Source: CAD feature listing. Evaluate the final solid. Frame: model axes, mm. A direction names the side the tool comes from. Round coordinates to 2 decimals unless told otherwise and drop trailing zeros. Loops run counter-clockwise (first coordinate to the right, second up) from the corner with the lowest first, then second, coordinate; pieces in that order, holes last. Notation, with made-up numbers: (80.25, -27.5) -> (85.25, -27.5) arc R18 cw to (85.25, 4.5) -> close; hole circle Ø3 at (-38, 61.5). An arc over 180 degrees is marked (long way). Return JSON: item names as keys, results as strings. Group by question number.
```python
from build123d import *

# Parameters (mm, degrees)
BOSS_EXTRUDE1_DEPTH = 1.524


with BuildPart() as part:
    # Sketch1 → Boss-Extrude1 (new body)
    with BuildSketch(Plane.XY):
        with BuildLine():
            Line((0, 36.766680051), (1.524, 36.766680051))
            Line((1.524, 36.766680051), (1.524, 38.982585825))
            Line((1.524, 38.982585825), (2.733148625, 38.375210755))
            Line((2.733148625, 38.375210755), (3.173163666, 37.740395602))
            ThreePointArc((3.173163666, 37.740395602), (2.76380149, 34.435260273), (2.111575724, 31.169360935))
            Line((2.111575724, 31.169360935), (3.752142818, 30.122391454))
            Line((3.752142818, 30.122391454), (1.811466825, 29.982342047))
            ThreePointArc((1.811466825, 29.982342047), (0.512131502, 25.907377193), (-1.167502988, 21.973875087))
            ThreePointArc((-1.167502988, 21.973875087), (-1.496079249, 21.518994961), (-1.833336721, 21.070513426))
            Line((-1.833336721, 21.070513426), (-0.732526116, 18.85197433))
            Line((-0.732526116, 18.85197433), (-2.63805659, 20.068036908))
            ThreePointArc((-2.63805659, 20.068036908), (-4.673990558, 17.880915718), (-6.922800397, 15.913333311))
            Line((-6.922800397, 15.913333311), (-6.657550745, 14.318385487))
            Line((-6.657550745, 14.318385487), (-7.787922662, 15.257015862))
            ThreePointArc((-7.787922662, 15.257015862), (-11.338183777, 13.037842353), (-15.16934542, 11.349267359))
            Line((-15.16934542, 11.349267359), (-15.723402455, 8.912532591))
            Line((-15.723402455, 8.912532591), (-16.164329399, 11.013577704))
            ThreePointArc((-16.164329399, 11.013577704), (-19.953116728, 10.084187136), (-23.831985363, 9.668189099))
            ThreePointArc((-23.831985363, 9.668189099), (-24.076075542, 9.604568952), (-24.319524306, 9.538536852))
            Line((-24.319524306, 9.538536852), (-24.695691572, 6.942894819))
            Line((-24.695691572, 6.942894819), (-25.27612991, 9.253711636))
            ThreePointArc((-25.27612991, 9.253711636), (-26.183331796, 8.945243362), (-27.078300937, 8.602901171))
            ThreePointArc((-27.078300937, 8.602901171), (-30.246868295, 7.97926726), (-32.962548086, 6.231748554))
            Line((-32.962548086, 6.231748554), (-32.532162923, 5.243855929))
            Line((-32.532162923, 5.243855929), (-33.480739201, 5.694007752))
            ThreePointArc((-33.480739201, 5.694007752), (-34.200835329, 4.756022574), (-34.785563978, 3.728186482))
            ThreePointArc((-34.785563978, 3.728186482), (-36.445037111, 2.053220727), (-37.942668533, 0.232105276))
            Line((-37.942668533, 0.232105276), (-37.938700484, 2.479305956))
            Line((-37.938700484, 2.479305956), (-35.209054914, 6.010902474))
            Line((-35.209054914, 6.010902474), (-36.41486015, 6.942894819))
            Line((-36.41486015, 6.942894819), (-37.934290003, 4.977067008))
            Line((-37.934290003, 4.977067008), (-37.932464483, 6.010902474))
            ThreePointArc((-37.932464483, 6.010902474), (-36.563778761, 7.575593862), (-34.971875943, 8.912532591))
            ThreePointArc((-34.971875943, 8.912532591), (-32.901550016, 9.116540541), (-30.910632492, 9.719960876))
            Line((-30.910632492, 9.719960876), (-30.910632492, 11.8237405))
            Line((-30.910632492, 11.8237405), (-29.95978759, 10.169722089))
            ThreePointArc((-29.95978759, 10.169722089), (-29.013670421, 10.741179379), (-28.13202331, 11.407812338))
            ThreePointArc((-28.13202331, 11.407812338), (-27.492889702, 11.44249827), (-26.85283117, 11.446965831))
            ThreePointArc((-26.85283117, 11.446965831), (-23.965434713, 11.605929088), (-21.115990345, 12.098873725))
            Line((-21.115990345, 12.098873725), (-20.706404595, 14.318385487))
            Line((-20.706404595, 14.318385487), (-20.019464899, 12.381448288))
            ThreePointArc((-20.019464899, 12.381448288), (-16.437841998, 13.695848714), (-13.099310966, 15.542435195))
            ThreePointArc((-13.099310966, 15.542435195), (-12.585951474, 15.59640554), (-12.076536587, 15.679755638))
            Line((-12.076536587, 15.679755638), (-11.031123121, 17.962204557))
            Line((-11.031123121, 17.962204557), (-11.249347571, 15.880665501))
            ThreePointArc((-11.249347571, 15.880665501), (-7.425610197, 18.149727188), (-5.157240456, 21.973875087))
            ThreePointArc((-5.157240456, 21.973875087), (-4.381951062, 24.278807565), (-3.708542129, 26.615537712))
            Line((-3.708542129, 26.615537712), (-5.157240456, 27.453082135))
            Line((-5.157240456, 27.453082135), (-3.412165634, 27.787336527))
            ThreePointArc((-3.412165634, 27.787336527), (-2.457151359, 32.712229886), (-1.951475295, 37.703313794))
            ThreePointArc((-1.951475295, 37.703313794), (-1.128983902, 38.484354747), (0, 38.375210755))
            Line((0, 38.375210755), (0, 36.766680051))
        make_face()
    extrude(amount=BOSS_EXTRUDE1_DEPTH)


solid = part.part
```
(1) Ray query, line 1 (X direction, y = 22, z = 1.1); line 2 (Y direction, x = -12.5, z = 0.5); line 3 (Y direction, x = -30.5, z = 1.35). Return the intervals inside material, ascending.
(2) Pin query (flat end, axial travel): pin 1 (0.5 mm diameter, centred on y = 38, z = 0.5, fed in from -X); pin 2 (0.8 mm diameter, centred on y = 11, z = 0.5, fed in from -X). Return the tip coordinate at first contact, or that it passes through.
(3) Cut plane A-A (y = 17). Return loops of the section in (x, z).
(4) Set-up query: faces 4 (the face through (-15.94, 9.95, 0.75)), 5 (the face through (-1.3, 20, 0.8)), 6 (the face through (-11.14, 16.94, 0.75)), 7 (the face through (-36.58, 7.56, 0.75)), 8 (the face through (-30.442, 11.008, 0.751)). Return all of +Z, -Z, +X, -X, +Y, -Y with unobstructed straight access to the full face (end or side cutting, diameter ignored); none if empty.
(5) Cut plane B-B (y = 35.5). Return loops of the section in (x, z).
(6) Mould query, pull axis Y, two halves, no side actions, for faces 1 (the face through (-4.297, 27.618, 0.751)), 2 (the face through (-33, 5.466, 0.751)), 3 (the face through (-6.792, 15.127, 0.751)). Classes: released by +Y, released by -Y, zero draft, split by the parting line, or undercut.
(7) Cut plane C-C (x = -10). Return loops of the section in (y, z).
Answers follow:
{
 "1": {"line 1": "-5.15 to -1.15", "line 2": "12.46 to 15.61", "line 3": "7.87 to 11.11"},
 "2": {"pin 1": "x = -1.93", "pin 2": "x = -30.91"},
 "3": {"outline": "(-11.47, 0) -> (-11.13, 0) -> (-11.13, 1.52) -> (-11.47, 1.52) -> close; (-8.84, 0) -> (-5.62, 0) -> (-5.62, 1.52) -> (-8.84, 1.52) -> close"},
 "4": {"face 4": "+Z, -Z, -Y", "face 5": "+Z, -Z, +X", "face 6": "+Z, -Z", "face 7": "+Z, -Z, -X, +Y", "face 8": "+Z, -Z, +Y"},
 "5": {"outline": "(-2.12, 0) -> (2.92, 0) -> (2.92, 1.52) -> (-2.12, 1.52) -> close"},
 "6": {"face 1": "released by +Y", "face 2": "released by -Y", "face 3": "undercut"},
 "7": {"outline": "(13.79, 0) -> (16.35, 0) -> (16.35, 1.52) -> (13.79, 1.52) -> close"}
}
